```python
from build123d import *

# Parameters (mm, degrees)
ESQUISSE1_W             = 100
ESQUISSE1_H             = 100
BOSS_EXTRU_1_DEPTH      = 3
ESQUISSE2_W             = 10
ESQUISSE2_H             = 20
BOSS_EXTRU_2_DEPTH      = 10
CHANFREIN1_SIZE         = 10
ESQUISSE3_R             = 1.525
ENL_V_MAT_EXTRU_1_DEPTH = 118.3413823
CHANFREIN2_SIZE         = 3
ESQUISSE4_W             = 5
ESQUISSE4_H             = 10
BOSS_EXTRU_3_DEPTH      = 10
ESQUISSE5_R             = 1.75
ENL_V_MAT_EXTRU_2_DEPTH = 10


with BuildPart() as part:
    # Esquisse1 → Boss.-Extru.1 (new body)
    with BuildSketch(Plane.XY):
        with Locations((50, 50)):
            Rectangle(ESQUISSE1_W, ESQUISSE1_H)
    extrude(amount=BOSS_EXTRU_1_DEPTH)

    # Esquisse2 → Boss.-Extru.2 (add)
    with BuildSketch(Plane.XY.offset(3)):
        with Locations((5.05, 50)):
            Rectangle(ESQUISSE2_W, ESQUISSE2_H)
        with Locations((94.95, 50)):
            Rectangle(ESQUISSE2_W, ESQUISSE2_H)
    extrude(amount=BOSS_EXTRU_2_DEPTH)

    # Chanfrein1
    chanfrein1_edges = [part.edges().sort_by_distance(p)[0] for p in [
        (94.95, 60, 13),
        (5.05, 60, 13),
    ]]
    chamfer(chanfrein1_edges, length=CHANFREIN1_SIZE - 0.0001)  # a hair under: the kernel refuses the full size

    # Esquisse3 → Enlèv. mat.-Extru.1 (cut, through all)
    with BuildSketch(Plane.XZ.offset(-40)):
        with Locations(Location((5.046227865, 8, 0), (0, 0, 270))):
            Circle(ESQUISSE3_R)
        with Locations(Location((94.95, 8, 0), (0, 0, 270))):
            Circle(ESQUISSE3_R)
    extrude(amount=-ENL_V_MAT_EXTRU_1_DEPTH, mode=Mode.SUBTRACT)

    # Chanfrein2
    chanfrein2_edges = [part.edges().sort_by_distance(p)[0] for p in [
        (50, 0, 0),
        (100, 50, 0),
        (50, 100, 0),
        (0, 50, 0),
    ]]
    chamfer(chanfrein2_edges, length=CHANFREIN2_SIZE - 0.0001)  # a hair under: the kernel refuses the full size

    # Esquisse4 → Boss.-Extru.3 (add)
    with BuildSketch(Plane.XY.offset(3)):
        with Locations((62.5, 94.95)):
            Rectangle(ESQUISSE4_W, ESQUISSE4_H)
    extrude(amount=BOSS_EXTRU_3_DEPTH)

    # Esquisse5 → Enlèv. mat.-Extru.2 (cut)
    with BuildSketch(Plane(origin=(65, 0, 0), x_dir=(0, 0, -1), z_dir=(1, 0, 0))):
        with Locations((-8.05, 94.95)):
            Circle(ESQUISSE5_R)
    extrude(amount=-ENL_V_MAT_EXTRU_2_DEPTH, mode=Mode.SUBTRACT)


solid = part.part
```
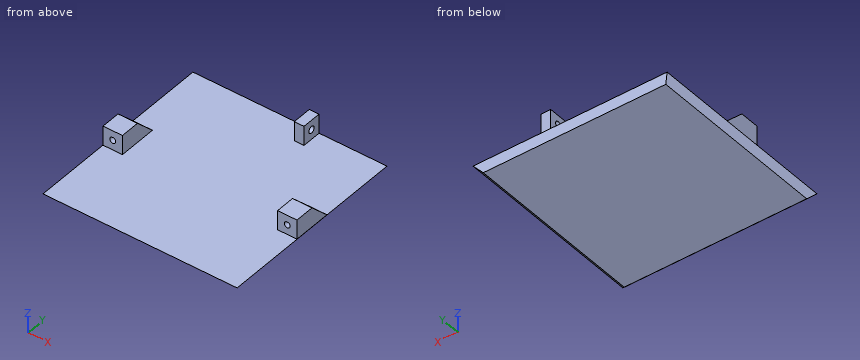
Work out the finished part from the listing and answer in its coordinate system (mm). Give positions to 0.01 mm unless a question says otherwise; leave off trailing zeros. Loops run counter-clockwise (first coordinate to the right, second up) from the corner with the lowest first, then second, coordinate; pieces in that order, holes last. Notation, with made-up numbers: (-17, 30) -> (19, 30) arc R28 ccw to (19, 53) -> close; hole circle Ø11 at (25, -31). An arc over 180 degrees is marked (long way). Use CSV: the item, a comma, the result in double quotes.
1. The part is cut by section B-B (z = 8.05). Write down the section's boundary in (x, y), then the cut area to 3 significant figures.
Found:
outline,"(0.05, 40) -> (3.52, 40) -> (3.52, 54.95) -> (0.05, 54.95) -> close; (6.57, 40) -> (10.05, 40) -> (10.05, 54.95) -> (6.57, 54.95) -> close; (60, 89.95) -> (65, 89.95) -> (65, 93.2) -> (60, 93.2) -> close; (60, 96.7) -> (65, 96.7) -> (65, 99.95) -> (60, 99.95) -> close; (89.95, 40) -> (93.43, 40) -> (93.43, 54.95) -> (89.95, 54.95) -> close; (96.47, 40) -> (99.95, 40) -> (99.95, 54.95) -> (96.47, 54.95) -> close"
area,"240 mm^2"
2. Flat-ended cylindrical pins translate along their axes: pin 1 Ø3 at (y, z) = (49.5, 8) entering from -X; pin 2 Ø5.5 at (x, z) = (62, 9) entering from +Y; pin 3 Ø5 at (x, z) = (97.5, 7) entering from -Y. Find the tip coordinate at first contact, or state that the pin passes through.
Found:
pin 1,"x = 0.05"
pin 2,"y = 99.95"
pin 3,"y = 40"
3. Straight lines are drawn through the part: line 1 (X direction, y = 50, z = 8) (3 decimals); line 2 (Z direction, x = 63.9, y = 94.95); line 3 (X direction, y = 43, z = 10). For each, find the intervals that lie inside material, in ascending order.
Found:
line 1,"0.05 to 3.521, 6.571 to 10.05, 89.95 to 93.425, 96.475 to 99.95"
line 2,"0 to 6.3, 9.8 to 13"
line 3,"0.05 to 10.05, 89.95 to 99.95"
